```python
from build123d import *

# Parameters (mm, degrees)
F0_R     = 3.302
F0_R_2   = 1.4605
F1_DEPTH = 4.7625


with BuildPart() as f1:
    # F0 (on Right) → F1 (new body)
    with BuildSketch(Plane.YZ):
        with BuildLine():
            Line((12.7, 12.7), (0, 12.7))
            Line((0, 12.7), (0, 0))
            Line((0, 0), (6.35, -20.6375))
            Line((6.35, -20.6375), (19.304, -20.6375))
            Line((19.304, -20.6375), (19.304, -25.4))
            Line((19.304, -25.4), (31.496, -25.4))
            Line((31.496, -25.4), (31.496, -20.6375))
            Line((31.496, -20.6375), (44.45, -20.6375))
            Line((44.45, -20.6375), (50.8, 0))
            Line((50.8, 0), (50.8, 12.7))
            Line((50.8, 12.7), (38.1, 12.7))
            ThreePointArc((38.1, 12.7), (33.609872, 14.559872), (31.75, 19.05))
            Line((31.75, 19.05), (31.75, 67.31))
            Line((31.75, 67.31), (19.05, 67.31))
            Line((19.05, 67.31), (19.05, 19.05))
            ThreePointArc((19.05, 19.05), (17.190128, 14.559872), (12.7, 12.7))
        make_face()
        with Locations((25.4, -9.2075)):
            Circle(F0_R, mode=Mode.SUBTRACT)
        with Locations((6.35, 6.35)):
            Circle(F0_R_2, mode=Mode.SUBTRACT)
        with Locations((44.45, 6.35)):
            Circle(F0_R_2, mode=Mode.SUBTRACT)
        with Locations((25.4, 60.96)):
            Circle(F0_R_2, mode=Mode.SUBTRACT)
    extrude(amount=F1_DEPTH)


solid = f1.part
```
Read the model definition and answer for the solid it produces. Units are mm, in the model's axes. A direction names the side the tool comes from. Coordinates: 2 decimals unless noted, no trailing zeros. Write each loop counter-clockwise with the first axis right and the second up, starting at its lowest first coordinate (ties: lowest second). Pieces come first, ordered by that corner, then holes. Notation, with made-up numbers: (-38.75, 87) -> (-1.75, 87) arc R18 ccw to (-1.75, 95) -> close; hole circle Ø7 at (-34, -30). An arc over 180 degrees is marked (long way). Return JSON: item names as keys, results as strings.
1. A cutting plane is placed at A-A (z = 60.96). Determine the outline of the cut face in (x, y).
Found:
{"outline": "(0, 19.05) -> (4.76, 19.05) -> (4.76, 23.94) -> (0, 23.94) -> close; (0, 26.86) -> (4.76, 26.86) -> (4.76, 31.75) -> (0, 31.75) -> close"}
2. A cutting plane is placed at C-C (z = 6.35). Determine the outline of the cut face in (x, y).
Found:
{"outline": "(0, 0) -> (4.76, 0) -> (4.76, 4.89) -> (0, 4.89) -> close; (0, 7.81) -> (4.76, 7.81) -> (4.76, 42.99) -> (0, 42.99) -> close; (0, 45.91) -> (4.76, 45.91) -> (4.76, 50.8) -> (0, 50.8) -> close"}
3. A tool of negligible diameter and unlimited length cuts with its end or side. For faces 5 (the face through (2, 31.75, 43)), 6 (the face through (2, 31.496, -23)), 7 (the face through (2, 13, -20.638)), 8 (the face through (2, 6, 12.7)), from which of +Z, -Z, +X, -X, +Y, -Y can it reach the whole face along a straight path? Write none if from no direction.
Found:
{"face 5": "+Z, +X, -X, +Y", "face 6": "-Z, +X, -X, +Y", "face 7": "-Z, +X, -X, -Y", "face 8": "+Z, +X, -X, -Y"}
4. Determine the mould class of faces 1 (the face through (2.35, 3.13, -10.17)), 2 (the face through (2.35, 23.94, 61.02)), 3 (the face through (2, 25, 67.31)), 4 (the face through (2, 19.05, 44)) for opening direction Z: pulls with the +Z half, pulls with the -Z half, needs draft (parallel to the pull), parting line crosses it, or undercut.
Found:
{"face 1": "pulls with the -Z half", "face 2": "undercut", "face 3": "pulls with the +Z half", "face 4": "needs draft"}
5. A cutting plane is placed at D-D (x = 2.2). Determine the outline of the cut face in (y, z).
Found:
{"outline": "(0, 0) -> (6.35, -20.64) -> (19.3, -20.64) -> (19.3, -25.4) -> (31.5, -25.4) -> (31.5, -20.64) -> (44.45, -20.64) -> (50.8, 0) -> (50.8, 12.7) -> (38.1, 12.7) arc R6.35 cw to (31.75, 19.05) -> (31.75, 67.31) -> (19.05, 67.31) -> (19.05, 19.05) arc R6.35 cw to (12.7, 12.7) -> (0, 12.7) -> close; hole circle Ø2.92 at (6.35, 6.35); hole circle Ø6.6 at (25.4, -9.21); hole circle Ø2.92 at (25.4, 60.96); hole circle Ø2.92 at (44.45, 6.35)"}
6. Find the intervals of material crossed by line 1 along Z through (x, y) = (1.95, 25.4); line 2 along Z through (x, y) = (4.5, 24.5); line 3 along Y through (x, z) = (3.6, 5.5), in increasing order. Write a range as from..to.
Found:
{"line 1": "-25.4..-12.51, -5.91..59.5, 62.42..67.31", "line 2": "-25.4..-12.38, -6.03..59.81, 62.11..67.31", "line 3": "0..5.16, 7.54..43.26, 45.64..50.8"}
7. Each of these flat-tipped pins is pushed along its axis until it touches: P1, Ø1.8, axis at y = 6.35, z = 6.35, coming from the -X side; P2, Ø1.4, axis at x = 2, y = 47.5, coming from the +Z side; P3, Ø2.5, axis at x = 2.5, y = 14, coming from the -Z side. Where does it stop, or does it pass through?
Found:
{"P1": "through", "P2": "z = 12.7", "P3": "z = -20.64"}
8. A cutting plane is placed at B-B (y = 25.4). Determine the outline of the cut face in (x, z), and give its area (3 significant figures).
Found:
{"outline": "(0, -25.4) -> (4.76, -25.4) -> (4.76, -12.51) -> (0, -12.51) -> close; (0, -5.91) -> (4.76, -5.91) -> (4.76, 59.5) -> (0, 59.5) -> close; (0, 62.42) -> (4.76, 62.42) -> (4.76, 67.31) -> (0, 67.31) -> close", "area": "396 mm2"}
